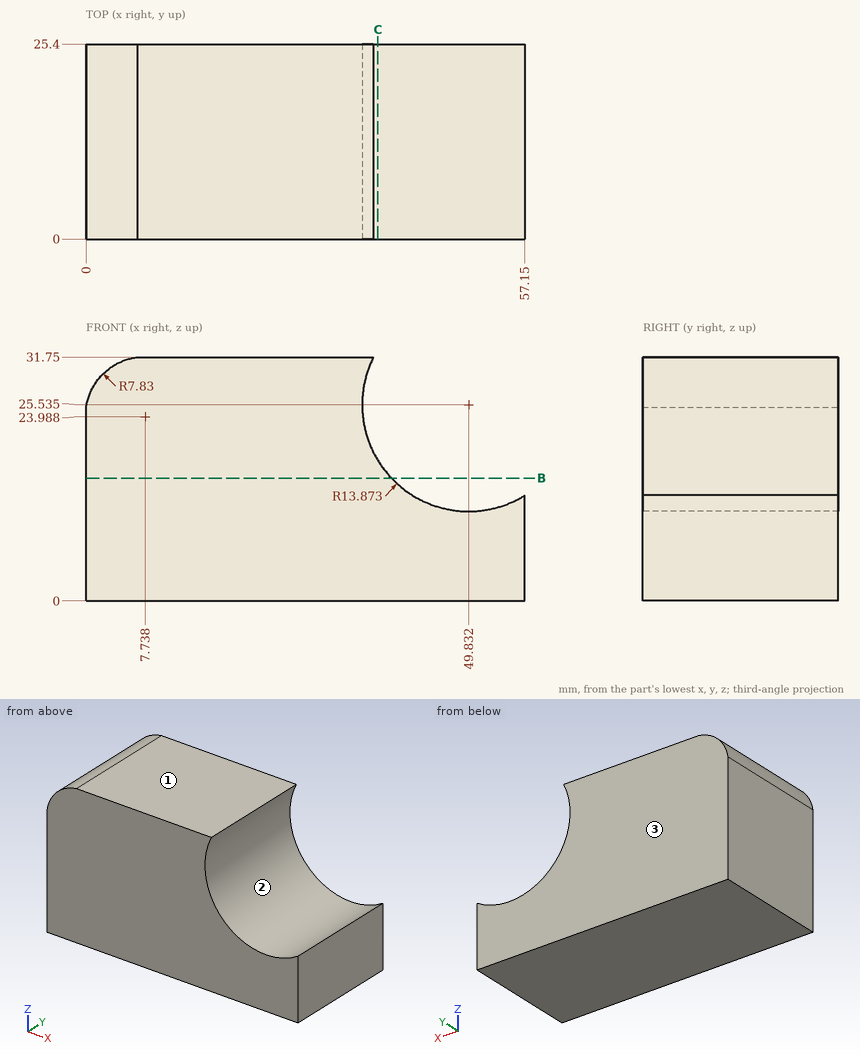
Input: dimensioned drawing with shaded views. Units: mm. Origin: part minimum x, y, z. Give positions to 0.01 mm unless a question says otherwise; leave off trailing zeros. Write each loop counter-clockwise with the first axis right and the second up, starting at its lowest first coordinate (ties: lowest second). Pieces come first, ordered by that corner, then holes. Notation, with made-up numbers: (18, 14.25) -> (28, 14.25) arc R23 ccw to (28, 48.25) -> close; hole circle Ø5 at (62.25, 26). An arc over 180 degrees is marked (long way). Answer as a JSON object with one key per item and string values.
1. Cut plane C-C on x = 38. Output: boundary loops of the cut face in (y, z).
Ans:
{"outline": "(0, 0) -> (25.4, 0) -> (25.4, 18.29) -> (0, 18.29) -> close"}
2. Mould query, pull axis Z, two halves, no side actions, for the marked faces 1, 2 and 3. Classes: pulls with the +Z half, pulls with the -Z half, needs draft (parallel to the pull), parting line crosses it, or undercut.
Ans:
{"face 1": "pulls with the +Z half", "face 2": "undercut", "face 3": "needs draft"}
3. Cut plane B-B on z = 16. Output: boundary loops of the cut face in (x, y) (1 decimal).
Ans:
{"outline": "(0, 0) -> (39.8, 0) -> (39.8, 25.4) -> (0, 25.4) -> close"}
4. Ray query, probe 1 along Z at (x, y) = (42.5, 18); probe 2 along X at (y, z) = (9.25, 22.5) (1 decimal); probe 3 along Z at (x, y) = (45, 15.25). Return the intervals inside material, ascending. Write a range as from..to.
Ans:
{"probe 1": "z = 0..13.76", "probe 2": "x = 0..36.3", "probe 3": "z = 0..12.53"}
